from build123d import *

# Parameters (mm, degrees)
F1_DEPTH     = 12.7
F3_R         = 1.75
F4_DEPTH     = 26.001
F5_R         = 1.75
F6_DEPTH     = 26.001
F8_DEPTH     = 3
F9_T4_ANGLE  = 188.2705145196
F9_S5_R      = 8
F9_T6_DEPTH  = 11
F9_T10_ANGLE = 188.2705145196
F9_S11_R     = 8
F9_T12_DEPTH = 11
F10_R        = 2.85
F10_R_2      = 1.75
F11_DEPTH    = 3
F12_R        = 2.85
F13_DEPTH    = 3
F14_T1_DEPTH = 37.7
F15_SIZE     = 2


# Not quite as in the source:
# - a fillet or chamfer that OpenCascade refuses, or shapes differently, is made with other operations: its cross-section is extruded or revolved along the edge and cut away or added


with BuildPart() as f1:
    # F0 (on Front) → F1 (new body)
    with BuildSketch(Plane.XZ):
        with BuildLine():
            Line((26, 0), (0, 0))
            Line((0, 0), (0, -26))
            Line((0, -26), (5.8, -26))
            Line((5.8, -26), (5.8, -17.0813202825))
            ThreePointArc((5.8, -17.0813202825), (3.8683903961, -11.8683903961), (5.8, -6.6554605098))
            Line((5.8, -6.6554605098), (5.8, -5.8))
            Line((5.8, -5.8), (6.6554605098, -5.8))
            ThreePointArc((6.6554605098, -5.8), (11.8683903961, -3.8683903961), (17.0813202825, -5.8))
            Line((17.0813202825, -5.8), (26, -5.8))
            Line((26, -5.8), (26, 0))
        make_face()
        with BuildLine():
            ThreePointArc((5.8, -6.6554605098), (6.2115361467, -6.2115361467), (6.6554605098, -5.8))
            Line((6.6554605098, -5.8), (5.8, -5.8))
            Line((5.8, -5.8), (5.8, -6.6554605098))
        make_face()
    extrude(amount=F1_DEPTH)

    # F3 (on face) → F4 (cut, through all)
    with BuildSketch(Plane.XY):
        with Locations((21.442, -6)):
            Circle(F3_R)
    extrude(amount=-F4_DEPTH, mode=Mode.SUBTRACT)

    # F5 (on face) → F6 (cut, through all)
    with BuildSketch(Plane(origin=(0, 0, 0), x_dir=(0, -1, 0), z_dir=(-1, 0, 0))):
        with Locations((6, -21.442)):
            Circle(F5_R)
    extrude(amount=-F6_DEPTH, mode=Mode.SUBTRACT)

    # F7 (on offset) → F8 (join, symmetric)
    with BuildSketch(Plane(origin=(0, -6, 0), x_dir=(-1, 0, 0), z_dir=(0, 1, 0))):
        with BuildLine():
            ThreePointArc((-3.8683903961, -11.8683903961), (-6.2115361467, -6.2115361467), (-11.8683903961, -3.8683903961))
            Line((-11.8683903961, -3.8683903961), (-11.8683903961, -5.8683903961))
            ThreePointArc((-11.8683903961, -5.8683903961), (-7.625749709, -7.625749709), (-5.8683903961, -11.8683903961))
            Line((-5.8683903961, -11.8683903961), (-3.8683903961, -11.8683903961))
        make_face()
    extrude(amount=F8_DEPTH, both=True)

    # F9: chamfer of 2 on 2 edges, made by hand


with BuildPart() as f9_tool2:
    # F9_s3 → F9_t4 (revolve)
    with BuildSketch(Plane(origin=(10.953058548, 0, -12.6602903485), x_dir=(0, 1, 0), z_dir=(0.6542755714, 0, -0.7562562242))):
        Polygon((-9, 9.2103462012), (-7, 7.2103462012), (-9, 7.2103462012), align=None)
    revolve(axis=Axis((11.8683903961, -9, -11.8683903961), (0, -1, 0)), revolution_arc=F9_T4_ANGLE)

    # F9_s5 → F9_t6 (intersect, symmetric)
    with BuildSketch(Plane.XZ.offset(8)):
        with Locations((11.8683903961, -11.8683903961)):
            Circle(F9_S5_R)
    extrude(amount=F9_T6_DEPTH, both=True, mode=Mode.INTERSECT)


with BuildPart() as f1_1:
    add(f1.part)

    # F9_t1: cut F9_tool2
    add(f9_tool2.part, mode=Mode.SUBTRACT)


with BuildPart() as f9_tool8:
    # F9_s9 → F9_t10 (revolve)
    with BuildSketch(Plane(origin=(10.953058548, 0, -12.6602903485), x_dir=(0, 1, 0), z_dir=(0.6542755714, 0, -0.7562562242))):
        Polygon((-3, 9.2103462012), (-5, 7.2103462012), (-3, 7.2103462012), align=None)
    revolve(axis=Axis((11.8683903961, -3, -11.8683903961), (0, -1, 0)), revolution_arc=F9_T10_ANGLE)

    # F9_s11 → F9_t12 (intersect, symmetric)
    with BuildSketch(Plane.XZ.offset(4)):
        with Locations((11.8683903961, -11.8683903961)):
            Circle(F9_S11_R)
    extrude(amount=F9_T12_DEPTH, both=True, mode=Mode.INTERSECT)


with BuildPart() as f1_2:
    add(f1_1.part)

    # F9_t7: cut F9_tool8
    add(f9_tool8.part, mode=Mode.SUBTRACT)

    # F10 (on face) → F11 (cut)
    with BuildSketch(Plane(origin=(0, 0, 0), x_dir=(0, -1, 0), z_dir=(-1, 0, 0))):
        with Locations((6, -21.442)):
            Circle(F10_R)
        with Locations((6, -21.442)):
            Circle(F10_R_2, mode=Mode.SUBTRACT)
    extrude(amount=-F11_DEPTH, mode=Mode.SUBTRACT)

    # F12 (on face) → F13 (cut)
    with BuildSketch(Plane.XY):
        with Locations((21.442, -6)):
            Circle(F12_R)
    extrude(amount=-F13_DEPTH, mode=Mode.SUBTRACT)

    # F14: fillet of radius 5 on 1 edges, made by hand

    # F14_s2 → F14_t1 (cut)
    with BuildSketch(Plane.XZ.offset(-12.5)):
        with BuildLine():
            ThreePointArc((5, 0), (1.4644660941, -1.4644660941), (0, -5))
            Line((0, -5), (0, 0))
            Line((0, 0), (5, 0))
        make_face()
    extrude(amount=F14_T1_DEPTH, mode=Mode.SUBTRACT)

    # F15
    f15_edges = [f1_2.edges().sort_by_distance(p)[0] for p in [
        (0, 0, -15.5),
        (1.464466, 0, -1.464466),
        (15.5, 0, 0),
    ]]
    chamfer(f15_edges, length=F15_SIZE)


solid = f1_2.part
Here's how the part is built. I have some questions about the finished solid (model axes, mm). A direction names the side the tool comes from. Give positions to 0.01 mm unless a question says otherwise; leave off trailing zeros. Loops run counter-clockwise (first coordinate to the right, second up) from the corner with the lowest first, then second, coordinate; pieces in that order, holes last. Notation, with made-up numbers: (-8, -11) -> (18, -11) arc R15 ccw to (18, -7) -> close; hole circle Ø5 at (-19.75, -7.5). An arc over 180 degrees is marked (long way). Answer as a JSON object with one key per item and string values. Group by question number.
Item 1: Imagine slicing it at D-D on x = 14.5. Write out the boundary of the cut face in (y, z).
Item 2: Imagine slicing it at B-B on y = -10. Write out the boundary of the cut face in (x, z).
Item 3: Will these pins go through, and if not, where does the flat tip stop? pin 1 (3 mm diameter, centred on y = -6, z = -21.442, fed in from +X); pin 2 (5 mm diameter, centred on y = -6, z = -21.442, fed in from -X); pin 3 (5.5 mm diameter, centred on x = 21.442, y = -6, fed in from -Z); pin 4 (2.5 mm diameter, centred on y = -4, z = -22.5, fed in from +X).
Item 4: Imagine slicing it at A-A on y = -6. Write out the boundary of the cut face in (x, z).
Item 5: I need wall thicknesses on L1, parallel to Z at x = 5.2, y = -6; L2, parallel to Z at x = 17.25, y = -5.5; L3, parallel to Z at x = 5.5, y = -9.5. Which ranges of each line are inside material? Lowest first, please.
Item 6: Thinking about a two-plate mould opening in X: for faces 4 (the conical face through (7.294, -4.458, -7.192)), 5 (the flat face through (11.868, -6, -5)), 6 (the cylindrical face through (2, -7, -1)), 7 (the flat face through (6, 0, -6)), which applies, pulls with the +X half, pulls with the -X half, needs draft (parallel to the pull), parting line crosses it, or undercut?
Item 7: Imagine slicing it at C-C on z = -4.25. Give the number of separate pieces and of enclosed holes in the cut face, then the cut area to 3 significant figures.
Item 8: On a 3-axis mill with a long thin cutter (end or side, diameter ignored), from which of +Z, -Z, +X, -X, +Y, -Y can I reach the whole of each face in a straight line? I mean faces 1 (the flat face through (3, -8, -21)), 2 (the flat face through (5, -6, -11.868)), 3 (the flat face through (5.8, -8, -21)). Say none if no direction works.
Answer list:
{
 "1": {"outline": "(-12.7, -4.31) -> (0, -4.31) -> (0, -2) -> (-2, 0) -> (-12.7, 0) -> close"},
 "2": {"outline": "(0, -26) -> (5.8, -26) -> (5.8, -17.08) arc R8 cw to (17.08, -5.8) -> (26, -5.8) -> (26, 0) -> (5, 0) arc R5 ccw to (0, -5) -> close"},
 "3": {"pin 1": "passes through", "pin 2": "stops at x = 3", "pin 3": "stops at z = -5.8", "pin 4": "stops at x = 5.8"},
 "4": {"outline": "(0, -26) -> (5.8, -26) -> (5.8, -23.19) -> (3, -23.19) -> (3, -24.29) -> (0, -24.29) -> close; (0, -18.59) -> (3, -18.59) -> (3, -19.69) -> (5.8, -19.69) -> (5.8, -17.08) arc R8 cw to (3.87, -11.87) -> (5.87, -11.87) arc R6 cw to (11.87, -5.87) -> (11.87, -3.87) arc R8 cw to (17.08, -5.8) -> (19.69, -5.8) -> (19.69, -3) -> (18.59, -3) -> (18.59, 0) -> (5, 0) arc R5 ccw to (0, -5) -> close; (23.19, -5.8) -> (26, -5.8) -> (26, 0) -> (24.29, 0) -> (24.29, -3) -> (23.19, -3) -> close"},
 "5": {"L1": "z = -26 to -23.19, -19.69 to -16.29, -11.87 to 0", "L2": "z = -5.8 to 0", "L3": "z = -26 to -16.71, -7.03 to 0"},
 "6": {"face 4": "undercut", "face 5": "undercut", "face 6": "pulls with the -X half", "face 7": "needs draft"},
 "7": {"separate pieces": "2", "enclosed holes": "1", "area": "269 mm2"},
 "8": {"face 1": "-X", "face 2": "+X, +Y, -Y", "face 3": "-Z, +X, +Y, -Y"}
}
